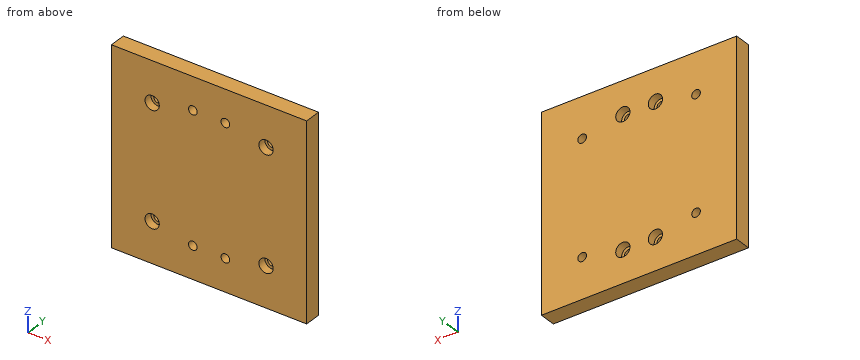
from build123d import *

# Parameters (mm, degrees)
SKETCH1_W                                        = 152.4
SKETCH1_H                                        = 152.4
BOSS_EXTRUDE1_DEPTH                              = 12.7
CBORE_FOR_1_4_SOCKET_HEAD_CAP_SCREW1_D           = 6.7564
CBORE_FOR_1_4_SOCKET_HEAD_CAP_SCREW1_CBORE_D     = 11.1125
CBORE_FOR_1_4_SOCKET_HEAD_CAP_SCREW1_CBORE_DEPTH = 6.35
CBORE_FOR_1_4_SOCKET_HEAD_CAP_SCREW2_D           = 6.7564
CBORE_FOR_1_4_SOCKET_HEAD_CAP_SCREW2_CBORE_D     = 11.1125
CBORE_FOR_1_4_SOCKET_HEAD_CAP_SCREW2_CBORE_DEPTH = 6.35


with BuildPart() as part:
    # Sketch1 → Boss-Extrude1 (new body)
    with BuildSketch(Plane(origin=(0, 0, 0), x_dir=(1, 0, 0), z_dir=(0, 1, 0))):
        Rectangle(SKETCH1_W, SKETCH1_H)
    extrude(amount=BOSS_EXTRUDE1_DEPTH)

    # CBORE for 1/4 Socket Head Cap Screw1 (through all)
    with Locations(Plane(origin=(0, 12.7, 0), x_dir=(1, 0, 0), z_dir=(0, 1, 0))):
        with Locations((-12.7, -50.8), (12.7, -50.8), (12.7, 50.8), (-12.7, 50.8)):
            CounterBoreHole(CBORE_FOR_1_4_SOCKET_HEAD_CAP_SCREW1_D / 2, CBORE_FOR_1_4_SOCKET_HEAD_CAP_SCREW1_CBORE_D / 2, CBORE_FOR_1_4_SOCKET_HEAD_CAP_SCREW1_CBORE_DEPTH)

    # CBORE for 1/4 Socket Head Cap Screw2 (through all)
    with Locations(Plane(origin=(0, 0, 0), x_dir=(-1, 0, 0), z_dir=(0, -1, 0))):
        with Locations((-44.45, -44.45), (-44.45, 44.45), (44.45, 44.45), (44.45, -44.45)):
            CounterBoreHole(CBORE_FOR_1_4_SOCKET_HEAD_CAP_SCREW2_D / 2, CBORE_FOR_1_4_SOCKET_HEAD_CAP_SCREW2_CBORE_D / 2, CBORE_FOR_1_4_SOCKET_HEAD_CAP_SCREW2_CBORE_DEPTH)


solid = part.part
Could you check a few things on this model? Use its own coordinates, in mm. Give positions to 0.01 mm unless a question says otherwise; leave off trailing zeros. Write each loop counter-clockwise with the first axis right and the second up, starting at its lowest first coordinate (ties: lowest second). Pieces come first, ordered by that corner, then holes. Notation, with made-up numbers: (34, 89.5) -> (62, 89.5) arc R23 ccw to (62, 109.5) -> close; hole circle Ø5 at (63, 16.25). An arc over 180 degrees is marked (long way). Answer as a JSON object with one key per item and string values.
Q1. Please list where these lines run through material, in increasing order: L1, parallel to Z at x = -12.7, y = 11.25; L2, parallel to Z at x = 44.45, y = 8.5; L3, parallel to X at y = 10.75, z = -50.8.
Taken from the geometry:
{"L1": "z = -76.2 to -56.36, -45.24 to 45.24, 56.36 to 76.2", "L2": "z = -76.2 to -47.83, -41.07 to 41.07, 47.83 to 76.2", "L3": "x = -76.2 to -18.26, -7.14 to 7.14, 18.26 to 76.2"}
Q2. Suppose I cut it at B-B on x = 12.7. Write out the boundary of the cut face in (y, z).
Taken from the geometry:
{"outline": "(0, -76.2) -> (12.7, -76.2) -> (12.7, -56.36) -> (6.35, -56.36) -> (6.35, -54.18) -> (0, -54.18) -> close; (0, -47.42) -> (6.35, -47.42) -> (6.35, -45.24) -> (12.7, -45.24) -> (12.7, 45.24) -> (6.35, 45.24) -> (6.35, 47.42) -> (0, 47.42) -> close; (0, 54.18) -> (6.35, 54.18) -> (6.35, 56.36) -> (12.7, 56.36) -> (12.7, 76.2) -> (0, 76.2) -> close"}
Q3. Will these pins go through, and if not, where does the flat tip stop? pin 1 Ø3.5 at (x, z) = (-11, 51.5) entering from +Y; pin 2 Ø13 at (x, z) = (-12.7, 50.8) entering from -Y.
Taken from the geometry:
{"pin 1": "stops at y = 6.35", "pin 2": "stops at y = 0"}
Q4. Suppose I cut it at A-A on y = 9.5. Count the separate pieces of the cut face and the enclosed holes in it, then the cut area to 3 significant figures.
Taken from the geometry:
{"separate pieces": "1", "enclosed holes": "8", "area": "22,700 mm²"}
Q5. Suppose I cut it at C-C on x = -13. Write out the boundary of the cut face in (y, z).
Taken from the geometry:
{"outline": "(0, -76.2) -> (12.7, -76.2) -> (12.7, -56.35) -> (6.35, -56.35) -> (6.35, -54.16) -> (0, -54.16) -> close; (0, -47.44) -> (6.35, -47.44) -> (6.35, -45.25) -> (12.7, -45.25) -> (12.7, 45.25) -> (6.35, 45.25) -> (6.35, 47.44) -> (0, 47.44) -> close; (0, 54.16) -> (6.35, 54.16) -> (6.35, 56.35) -> (12.7, 56.35) -> (12.7, 76.2) -> (0, 76.2) -> close"}
